Could you check a few things on this model? Use its own coordinates, in mm. Round coordinates to 2 decimals unless told otherwise and drop trailing zeros. Write each loop counter-clockwise with the first axis right and the second up, starting at its lowest first coordinate (ties: lowest second). Pieces come first, ordered by that corner, then holes. Notation, with made-up numbers: (26.5, 4) -> (56.5, 4) arc R21 ccw to (56.5, 32) -> close; hole circle Ø1 at (53, -37). An arc over 180 degrees is marked (long way). One line per question, with ' | ' between items. Start each with the question number.
1. Thinking about a two-plate mould opening in Y: for faces 1 (the flat face through (-49, 43, 0)), 2 (the cylindrical face through (1.802, 59.904, 7.535)), 3 (the flat face through (-49, -5.405, 5)), which applies, released by +Y, released by -Y, zero draft, split by the parting line, or undercut?
2. Imagine slicing it at A-A, the plane x = 18.5. List the corners of the cut face in (y, z) for me, and give its area (3 significant figures).
3. If I drill on line 1 along X through (y, z) = (54.5, 9); line 2 along X through (y, z) = (51, 7.5); line 3 along Y through (x, z) = (-19.5, 9.75), over which ranges is the centre line in solid material (lowest first)? Write a range as [from, to].
4. For pin 1 Ø18.5 at (x, y) = (0.07, 52.09) entering from -Z, with a flat end and sliding along its axis, tell me the tip position at first contact or that it passes through.
from build123d import *

# Parameters (mm, degrees)
F0_W           = 210
F0_H           = 100
F1_DEPTH       = 10
F2_D           = 5
F2_CSINK_D     = 10
F2_CSINK_ANGLE = 90
F3_D           = 16
F3_CSINK_D     = 26
F3_CSINK_ANGLE = 90
F4_SIZE        = 4


with BuildPart() as f1:
    # F0 (on Top) → F1 (new body)
    with BuildSketch(Plane.XY):
        with Locations((-47.4317967892, 44.5945628711)):
            Rectangle(F0_W, F0_H)
    extrude(amount=F1_DEPTH)

    # F2 (through all)
    with Locations(Plane(origin=(0, 0, 0), x_dir=(1, 0, 0), z_dir=(0, 0, -1))):
        with Locations((30.0682032108, -44.5945628711), (-142.4317967892, -44.5945628711)):
            CounterSinkHole(F2_D / 2, F2_CSINK_D / 2, counter_sink_angle=F2_CSINK_ANGLE)

    # F3 (through all)
    with Locations(Plane(origin=(0, 0, 0), x_dir=(1, 0, 0), z_dir=(0, 0, -1))):
        with Locations((-114.9317967892, -52.0945628711), (0.0682032108, -52.0945628711)):
            CounterSinkHole(F3_D / 2, F3_CSINK_D / 2, counter_sink_angle=F3_CSINK_ANGLE)

    # F4
    f4_edges = [f1.edges().sort_by_distance(p)[0] for p in [
        (-47.431797, 94.594563, 0),
        (-47.431797, 94.594563, 10),
    ]]
    chamfer(f4_edges, length=F4_SIZE)


solid = f1.part
Geometry results:
1) face 1: zero draft | face 2: undercut | face 3: released by -Y
2) outline: (-5.41, 0) -> (90.59, 0) -> (94.59, 4) -> (94.59, 6) -> (90.59, 10) -> (-5.41, 10) -> close | area: 984 mm2
3) line 1: x = [-152.43, -122.56], [-107.3, -7.56], [7.7, 57.57] | line 2: x = [-152.43, -122.86], [-107.01, -7.86], [7.99, 57.57] | line 3: y = [-5.41, 90.84]
4) pin 1: stops at z = 3.75
